For this review, take the finished solid that the model builds, in its own axes (mm). A direction names the side the tool comes from. Coordinates: 2 decimals unless noted, no trailing zeros. Order: outer loops, then holes, each group sorted by start corner. A loop starts at its lowest first (then second) coordinate and runs counter-clockwise, first axis right, second up. Notation, with made-up numbers: M 53.5,52 L 60.5,52 A15 ccw 60.5,65 Z; hole C 25.5,46.25 d1. An arc over 180 degrees is marked long. Use one line per item in the form item = value. Start each with the question number.
```python
from build123d import *

# Parameters (mm, degrees)
F0_W        = 25.4
F0_H        = 50.8
F1_DEPTH    = 228.6
F2_W        = 21.971
F2_H        = 47.371
F3_DEPTH    = 457.201
F4_R        = 1.5875
F5_DEPTH    = 25.401
F6_R        = 1.5875
F7_DEPTH    = 25.401
F8_T1_DEPTH = 152.4
F9_T1_DEPTH = 152.4


# Not quite as in the source:
# - a fillet or chamfer that OpenCascade refuses, or shapes differently, is made with other operations: its cross-section is extruded or revolved along the edge and cut away or added


with BuildPart() as f1:
    # F0 (on Right) → F1 (new body, symmetric)
    with BuildSketch(Plane.YZ):
        Rectangle(F0_W, F0_H)
    extrude(amount=F1_DEPTH, both=True)

    # F2 (on face) → F3 (cut, through all)
    with BuildSketch(Plane.YZ.offset(228.6)):
        Rectangle(F2_W, F2_H)
    extrude(amount=-F3_DEPTH, mode=Mode.SUBTRACT)

    # F4 (on face) → F5 (cut, through all)
    with BuildSketch(Plane.XZ.offset(12.7)):
        with Locations((-210.82, 0)):
            Circle(F4_R)
        Circle(F4_R)
    extrude(amount=-F5_DEPTH, mode=Mode.SUBTRACT)

    # F6 (on face) → F7 (cut, through all)
    with BuildSketch(Plane.XZ.offset(12.7)):
        with Locations((210.82, 0)):
            Circle(F6_R)
    extrude(amount=-F7_DEPTH, mode=Mode.SUBTRACT)

    # F8: fillet of radius 25.4 on 2 edges, made by hand

    # F8_s2 → F8_t1 (cut)
    with BuildSketch(Plane.XZ.offset(-76.2)):
        with BuildLine():
            ThreePointArc((-228.6, 0), (-221.1605122421, -17.9605122421), (-203.2, -25.4))
            Line((-203.2, -25.4), (-228.6, -25.4))
            Line((-228.6, -25.4), (-228.6, 0))
        make_face()
        with BuildLine():
            ThreePointArc((-228.6, 0), (-221.1605122421, 17.9605122421), (-203.2, 25.4))
            Line((-203.2, 25.4), (-228.6, 25.4))
            Line((-228.6, 25.4), (-228.6, 0))
        make_face()
    extrude(amount=F8_T1_DEPTH, mode=Mode.SUBTRACT)

    # F9: fillet of radius 25.4 on 2 edges, made by hand

    # F9_s2 → F9_t1 (cut)
    with BuildSketch(Plane.XZ.offset(-76.2)):
        with BuildLine():
            ThreePointArc((203.2, 25.4), (221.1605122421, 17.9605122421), (228.6, 0))
            Line((228.6, 0), (228.6, 25.4))
            Line((228.6, 25.4), (203.2, 25.4))
        make_face()
        with BuildLine():
            ThreePointArc((228.6, 0), (221.1605122421, -17.9605122421), (203.2, -25.4))
            Line((203.2, -25.4), (228.6, -25.4))
            Line((228.6, -25.4), (228.6, 0))
        make_face()
    extrude(amount=F9_T1_DEPTH, mode=Mode.SUBTRACT)


solid = f1.part
```
1. Consider section A-A, the plane y = 1.75. Write out the cut boundary in (x, z).
2. To check wall thickness, follow line 1 (Z direction, x = 45, y = 9.5); line 2 (Y direction, x = 79.5, z = -9); line 3 (Z direction, x = 0, y = -11.45). State the ranges of each line that lie inside material, in increasing order.
3. Tool access review of faces 4 (the flat face through (3, 0, 25.4)), 5 (the flat face through (3, 10.986, 0)): name each direction out of +Z, -Z, +X, -X, +Y, -Y from which nothing blocks a thin tool from reaching the whole face with its end or side.
4. Consider section C-C, the plane x = -108.5. Write out the cut boundary in (y, z), plus the area to 3 significant figures.
5. For pin 1 Ø2 at (y, z) = (-9.5, 9) entering from +X; pin 2 Ø3.5 at (x, z) = (210.82, 0) entering from -Y; pin 3 Ø3 at (y, z) = (10, 7.5) entering from -X, all flat-tipped, find the tip position at first contact; note any pin that passes through.
6. Consider section B-B, the plane z = -17. Write out the cut boundary in (x, y), plus the area to 3 significant figures.
7. The part is to be moulded in two halves that separate along Y. For faces 1 (the flat face through (3, 0, -23.686)), 2 (the flat face through (3, 0, -25.4)), 3 (the flat face through (3, -12.7, 0)), say which applies: pulls with the +Y half, pulls with the -Y half, needs draft (parallel to the pull), parting line crosses it, or undercut.
Answers follow:
q1.outline = M -212.37,-23.69 A25.4 ccw -203.2,-25.4 L 203.2,-25.4 A25.4 ccw 212.37,-23.69 Z; M -212.37,23.69 L 212.37,23.69 A25.4 ccw 203.2,25.4 L -203.2,25.4 A25.4 ccw Z
q2.line_1 = -25.4 to -23.69, 23.69 to 25.4
q2.line_2 = -12.7 to -10.99, 10.99 to 12.7
q2.line_3 = -25.4 to -1.59, 1.59 to 25.4
q3.face_4 = +Z, +X, -X, +Y, -Y
q3.face_5 = +X, -X
q4.outline = M -12.7,-25.4 L 12.7,-25.4 L 12.7,25.4 L -12.7,25.4 Z; hole M -10.99,-23.69 L 10.99,-23.69 L 10.99,23.69 L -10.99,23.69 Z
q4.area = 250 mm²
q5.pin_1 = through
q5.pin_2 = -12.7
q5.pin_3 = -227.79
q6.outline = M -222.07,-12.7 L 222.07,-12.7 L 222.07,-10.99 L -222.07,-10.99 Z; M -222.07,10.99 L 222.07,10.99 L 222.07,12.7 L -222.07,12.7 Z
q6.area = 1,520 mm²
q7.face_1 = undercut
q7.face_2 = needs draft
q7.face_3 = pulls with the -Y half
